```python
from build123d import *

# Parameters (mm, degrees)
SKETCH_1_W          = 70
SKETCH_1_H          = 70
EXTRUDE_1_DEPTH     = 2.5
SKETCH_2_W          = 30
SKETCH_2_H          = 30
CUT_EXTRUDE_1_DEPTH = 1.7
SKETCH_3_R          = 2.6
CUT_EXTRUDE_2_DEPTH = 3
EXTRUDE_2_DEPTH     = 2
SKETCH_6_R          = 1.6
EXTRUDE_3_DEPTH     = 0.3


with BuildPart() as part:
    # 草图1 → 凸台-拉伸1 (new body)
    with BuildSketch(Plane.XY):
        with BuildLine():
            Line((-2, 17), (0, 17))
            Line((0, 17), (0, 53))
            Line((0, 53), (-2, 53))
            ThreePointArc((-2, 53), (-4.121320344, 52.121320344), (-5, 50))
            Line((-5, 50), (-5, 20))
            ThreePointArc((-5, 20), (-4.121320344, 17.878679656), (-2, 17))
        make_face()
        with Locations((35, 35)):
            Rectangle(SKETCH_1_W, SKETCH_1_H)
        with BuildLine():
            Line((70, 53), (70, 17))
            Line((70, 17), (72, 17))
            ThreePointArc((72, 17), (74.121320344, 17.878679656), (75, 20))
            Line((75, 20), (75, 50))
            ThreePointArc((75, 50), (74.121320344, 52.121320344), (72, 53))
            Line((72, 53), (70, 53))
        make_face()
    extrude(amount=EXTRUDE_1_DEPTH)

    # 草图2 → 切除-拉伸1 (cut)
    with BuildSketch(Plane.XY.offset(2.5)):
        with Locations((35, 35)):
            Rectangle(SKETCH_2_W, SKETCH_2_H)
    extrude(amount=-CUT_EXTRUDE_1_DEPTH, mode=Mode.SUBTRACT)

    # 草图3 → 切除-拉伸2 (cut)
    with BuildSketch(Plane.XY.offset(2.5)):
        with Locations((8, 62)):
            Circle(SKETCH_3_R)
        with Locations((62, 62)):
            Circle(SKETCH_3_R)
        with Locations((8, 8)):
            Circle(SKETCH_3_R)
        with Locations((62, 8)):
            Circle(SKETCH_3_R)
    extrude(amount=-CUT_EXTRUDE_2_DEPTH, mode=Mode.SUBTRACT)

    # 草图4 → 凸台-拉伸2 (add)
    with BuildSketch(Plane.XY):
        with BuildLine():
            Line((20, 44), (20, 50))
            Line((20, 50), (26, 50))
            ThreePointArc((26, 50), (24.242640687, 45.757359313), (20, 44))
        make_face()
        with BuildLine():
            Line((50, 44), (50, 50))
            Line((50, 50), (44, 50))
            ThreePointArc((44, 50), (45.757359313, 45.757359313), (50, 44))
        make_face()
        with BuildLine():
            Line((50, 20), (44, 20))
            ThreePointArc((44, 20), (45.757359313, 24.242640687), (50, 26))
            Line((50, 26), (50, 20))
        make_face()
        with BuildLine():
            Line((20, 26), (20, 20))
            Line((20, 20), (26, 20))
            ThreePointArc((26, 20), (24.242640687, 24.242640687), (20, 26))
        make_face()
    extrude(amount=EXTRUDE_2_DEPTH)

    # 草图6 → 凸台-拉伸3 (add)
    with BuildSketch(Plane.XY.offset(2)):
        with Locations((22.5, 47.5)):
            Circle(SKETCH_6_R)
        with Locations((47.5, 47.5)):
            Circle(SKETCH_6_R)
        with Locations((47.5, 22.5)):
            Circle(SKETCH_6_R)
        with Locations((22.5, 22.5)):
            Circle(SKETCH_6_R)
        Polygon((20.1, 45.5), (20.7, 45.5), (20.7, 46.1), (21.3, 46.1), (21.3, 45.5), (21.9, 45.5), (21.9, 44.9), (21.3, 44.9), (21.3, 44.3), (20.7, 44.3), (20.7, 44.9), (20.1, 44.9), align=None)
    extrude(amount=EXTRUDE_3_DEPTH)


solid = part.part
```
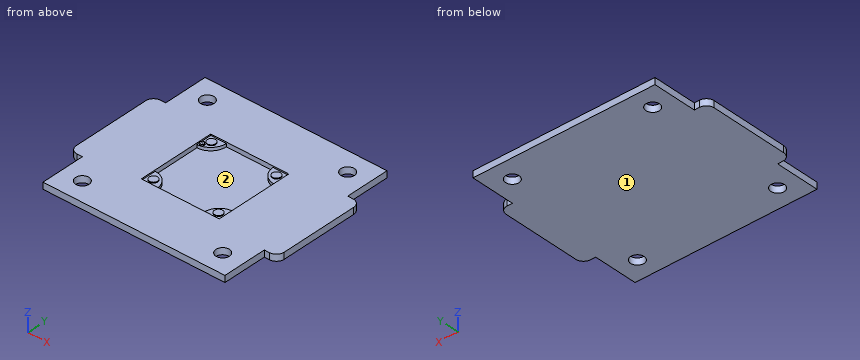
Geometry: final body of the model. Coordinates: model frame, mm. Face numbers are marked on the shaded views. Coordinates: 2 decimals unless noted, no trailing zeros. Order: outer loops, then holes, each group sorted by start corner. A loop starts at its lowest first (then second) coordinate and runs counter-clockwise, first axis right, second up.
Item 1: Section query D-D (x = 35.5). Output: boundary loops of the cut face in (y, z).
Answer:
outline: (0, 0) - (70, 0) - (70, 2.5) - (50, 2.5) - (50, 0.8) - (20, 0.8) - (20, 2.5) - (0, 2.5) - close
Item 2: Material intervals for line 1 along Y through (x, z) = (8, 1.1); line 2 along X through (y, z) = (39, 2.35); line 3 along Y through (x, z) = (41, 2.1), sorted ascending.
Answer:
line 1: y = 0 to 5.4, 10.6 to 59.4, 64.6 to 70
line 2: x = -5 to 20, 50 to 75
line 3: y = 0 to 20, 50 to 70
Item 3: Section query A-A (z = 1.6). Output: boundary loops of the cut face in (x, y).
Answer:
outline: (-5, 20) arc R3 ccw to (-2, 17) - (0, 17) - (0, 0) - (70, 0) - (70, 17) - (72, 17) arc R3 ccw to (75, 20) - (75, 50) arc R3 ccw to (72, 53) - (70, 53) - (70, 70) - (0, 70) - (0, 53) - (-2, 53) arc R3 ccw to (-5, 50) - close; hole circle Ø5.2 at (8, 8); hole circle Ø5.2 at (8, 62); hole (20, 26) arc R6 cw to (26, 20) - (44, 20) arc R6 cw to (50, 26) - (50, 44) arc R6 cw to (44, 50) - (26, 50) arc R6 cw to (20, 44) - close; hole circle Ø5.2 at (62, 8); hole circle Ø5.2 at (62, 62)
Item 4: Section query B-B (x = 62). Output: boundary loops of the cut face in (y, z).
Answer:
outline: (0, 0) - (5.4, 0) - (5.4, 2.5) - (0, 2.5) - close; (10.6, 0) - (59.4, 0) - (59.4, 2.5) - (10.6, 2.5) - close; (64.6, 0) - (70, 0) - (70, 2.5) - (64.6, 2.5) - close
Item 5: Contact query for flat-ended pins moving along their axis: P1, Ø0.9, axis at x = 20.5, y = 45.5, coming from the +Z side; P2, Ø1.5, axis at y = 13.5, z = 0.5, coming from the +X side; P3, Ø1, axis at x = 71, z = 0.5, coming from the +Y side. Output: stop coordinate, or through.
Answer:
P1: stops at z = 2.3
P2: stops at x = 70
P3: stops at y = 53
Item 6: Draft query along Y for the marked faces 1 and 2. Return one class per face: released by +Y, released by -Y, zero draft, split by the parting line, or undercut.
Answer:
face 1: zero draft
face 2: undercut
